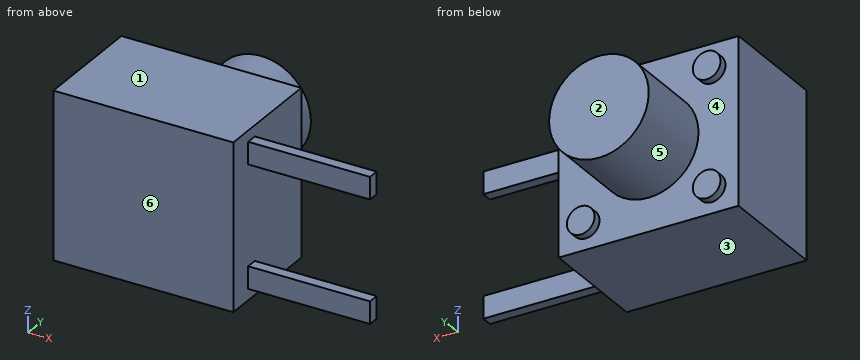
from build123d import *

# Parameters (mm, degrees)
SKETCH_1_W      = 6.5
SKETCH_1_H      = 6
EXTRUDE_1_DEPTH = 4.1
SKETCH_1_3_R    = 1.8
EXTRUDE_2_DEPTH = 7.1
EXTRUDE_START   = 4.1
SKETCH_1_4_R    = 0.5
EXTRUDE_3_DEPTH = 0.3
SKETCH_2_W      = 0.8
SKETCH_2_H      = 0.4
EXTRUDE_4_DEPTH = 4.4


with BuildPart() as part:
    # 草图1 → 凸台-拉伸1 (new body)
    with BuildSketch(Plane(origin=(0, 0, 0), x_dir=(1, 0, 0), z_dir=(0, 1, 0))):
        Rectangle(SKETCH_1_W, SKETCH_1_H)
    extrude(amount=EXTRUDE_1_DEPTH)

    # 草图1<3> → 凸台-拉伸2 (add)
    with BuildSketch(Plane(origin=(0, 0, 0), x_dir=(1, 0, 0), z_dir=(0, 1, 0))):
        with Locations(Location((0, 0, 0), (0, 0, 90))):
            Circle(SKETCH_1_3_R)
    extrude(amount=EXTRUDE_2_DEPTH)

    # 草图1<4> → 凸台-拉伸3 (add)
    with BuildSketch(Plane(origin=(0, 0, 0), x_dir=(1, 0, 0), z_dir=(0, 1, 0)).offset(EXTRUDE_START)):
        with Locations(Location((-2.275, 2.1, 0), (0, 0, 90))):
            Circle(SKETCH_1_4_R)
        with Locations(Location((-2.275, -2.1, 0), (0, 0, 90))):
            Circle(SKETCH_1_4_R)
        with Locations(Location((2.275, -2.1, 0), (0, 0, 90))):
            Circle(SKETCH_1_4_R)
        with Locations(Location((2.275, 2.1, 0), (0, 0, 90))):
            Circle(SKETCH_1_4_R)
    extrude(amount=EXTRUDE_3_DEPTH)

    # 草图2 → 凸台-拉伸4 (add)
    with BuildSketch(Plane(origin=(3.25, 0, 0), x_dir=(0, 0, -1), z_dir=(1, 0, 0))):
        with Locations((-2.2, 1.1)):
            Rectangle(SKETCH_2_W, SKETCH_2_H)
        with Locations((2.2, 1.1)):
            Rectangle(SKETCH_2_W, SKETCH_2_H)
    extrude(amount=EXTRUDE_4_DEPTH)


solid = part.part
Input: part model. Units: mm. Frame: model coordinates. Face numbers are marked on the shaded views. A direction names the side the tool comes from. Round coordinates to 2 decimals unless told otherwise and drop trailing zeros. Order: outer loops, then holes, each group sorted by start corner. A loop starts at its lowest first (then second) coordinate and runs counter-clockwise, first axis right, second up.
1. Cut plane B-B, the plane z = 2.1. Output: boundary loops of the cut face in (x, y) (3 decimals).
The answers:
outline: (-3.25, 0) - (3.25, 0) - (3.25, 0.9) - (7.65, 0.9) - (7.65, 1.3) - (3.25, 1.3) - (3.25, 4.1) - (2.775, 4.1) - (2.775, 4.4) - (1.775, 4.4) - (1.775, 4.1) - (-1.775, 4.1) - (-1.775, 4.4) - (-2.775, 4.4) - (-2.775, 4.1) - (-3.25, 4.1) - close
2. Pin query (flat end, axial travel): P1, Ø0.5, axis at x = -2.5, z = 2, coming from the +Y side; P2, Ø3.5, axis at y = 2, z = -0.5, coming from the +X side; P3, Ø1.5, axis at y = 4, z = 0, coming from the +X side; P4, Ø3, axis at y = 6.5, z = 0, coming from the +X side. Return the tip coordinate at first contact, or that it passes through.
The answers:
P1: stops at y = 4.4
P2: stops at x = 7.65
P3: stops at x = 3.25
P4: stops at x = 1.8
3. Cut plane C-C, the plane x = 0. Output: boundary loops of the cut face in (y, z).
The answers:
outline: (0, -3) - (4.1, -3) - (4.1, -1.8) - (7.1, -1.8) - (7.1, 1.8) - (4.1, 1.8) - (4.1, 3) - (0, 3) - close
4. Set-up query: the marked faces 5 and 6. Return all of +Z, -Z, +X, -X, +Y, -Y with unobstructed straight access to the full face (end or side cutting, diameter ignored); none if empty.
The answers:
face 5: +Y
face 6: +Z, -Z, +X, -X, -Y
5. Material intervals for line 1 (Z direction, x = 3.75, y = 1); line 2 (X direction, y = 1.5, z = -1.3); line 3 (X direction, y = 5.75, z = 0), sorted ascending.
The answers:
line 1: z = -2.6 to -1.8, 1.8 to 2.6
line 2: x = -3.25 to 3.25
line 3: x = -1.8 to 1.8
6. Mould query, pull axis Z, two halves, no side actions, for the marked faces 1, 2, 3 and 4. Classes: released by +Z, released by -Z, zero draft, split by the parting line, or undercut.
The answers:
face 1: released by +Z
face 2: zero draft
face 3: released by -Z
face 4: undercut
7. Cut plane A-A, the plane x = 5.25. Output: boundary loops of the cut face in (y, z), then the cut area to 3 significant figures.
The answers:
outline: (0.9, -2.6) - (1.3, -2.6) - (1.3, -1.8) - (0.9, -1.8) - close; (0.9, 1.8) - (1.3, 1.8) - (1.3, 2.6) - (0.9, 2.6) - close
area: 0.640 mm2
8. Cut plane D-D, the plane y = 1.75. Output: boundary loops of the cut face in (x, z).
The answers:
outline: (-3.25, -3) - (3.25, -3) - (3.25, 3) - (-3.25, 3) - close
